Read the model definition and answer for the solid it produces. Units are mm, in the model's axes. Coordinates: 2 decimals unless noted, no trailing zeros. Order: outer loops, then holes, each group sorted by start corner. A loop starts at its lowest first (then second) coordinate and runs counter-clockwise, first axis right, second up. Notation, with made-up numbers: (-8.5, -25) -> (-2.5, -25) arc R35 ccw to (-2.5, 10) -> close; hole circle Ø4 at (39, -27). An arc over 180 degrees is marked (long way). Answer as a JSON object with one key per item and string values. Group by question number.
1) Section A-A on x = -12.5 is taken. Determine the outline of the cut face in (y, z), and give its area (4 significant figures).
2) Section C-C on y = 60 is taken. Determine the outline of the cut face in (x, z), and give its area (3 significant figures).
3) Consider L1, parallel to Y at x = 41, z = 0; L2, parallel to Y at x = -4, z = -0.75; L3, parallel to X at y = 7, z = 0.75. Determine where each line is inside the solid, lowest interval first.
4) Section B-B on y = 30 is taken. Determine the outline of the cut face in (x, z).
5) Section D-D on z = -0.5 is taken. Count the separate pieces of the cut face and the enclosed holes in it, and give its area (3 significant figures).
6) Given pin 1 (4 mm diameter, centred on x = -4, y = 4, fed in from +Z), flat-ended and moving along its own axis, determine where the tip first touches the part or whether it passes through.
7) Determine the mould class of faces 1 (the flat face through (-1, 0, 0)), 2 (the cylindrical face through (-2.17, 50.24, 0.07)), 3 (the flat face through (60, 59, 0)) for opening direction Y: released by +Y, released by -Y, zero draft, split by the parting line, or undercut.
from build123d import *

# Parameters (mm, degrees)
SKETCH1_W           = 120
SKETCH1_H           = 10
BOSS_EXTRUDE1_DEPTH = 120
SKETCH2_R           = 2.25
SKETCH2_R_2         = 2.75
SKETCH2_R_3         = 10
SKETCH2_R_4         = 3.25
CUT_EXTRUDE1_DEPTH  = 10


with BuildPart() as part:
    # Sketch1 → Boss-Extrude1 (new body)
    with BuildSketch(Plane(origin=(0, 0, 0), x_dir=(1, 0, 0), z_dir=(0, 1, 0))):
        Rectangle(SKETCH1_W, SKETCH1_H)
    extrude(amount=BOSS_EXTRUDE1_DEPTH)

    # Sketch2 → Cut-Extrude1 (cut)
    with BuildSketch(Plane.XY.offset(5)):
        with Locations((-17.5, 77.5)):
            Circle(SKETCH2_R)
        with Locations((-12.5, 47.5)):
            Circle(SKETCH2_R)
        with Locations((12.5, 47.5)):
            Circle(SKETCH2_R)
        with Locations((17.5, 77.5)):
            Circle(SKETCH2_R)
        with Locations((55, 5)):
            Circle(SKETCH2_R_2)
        with Locations((55, 115)):
            Circle(SKETCH2_R_2)
        with Locations((0, 60)):
            Circle(SKETCH2_R_3)
        with Locations((-41, 90)):
            Circle(SKETCH2_R_2)
        with Locations((-41, 60)):
            Circle(SKETCH2_R_2)
        with Locations((-41, 30)):
            Circle(SKETCH2_R_2)
        with Locations((41, 30)):
            Circle(SKETCH2_R_2)
        with Locations((41, 60)):
            Circle(SKETCH2_R_2)
        with Locations((-4, 116)):
            Circle(SKETCH2_R_4)
        with Locations((4, 116)):
            Circle(SKETCH2_R_4)
        with Locations((41, 90)):
            Circle(SKETCH2_R_2)
        with Locations((-4, 4)):
            Circle(SKETCH2_R_4)
        with Locations((4, 4)):
            Circle(SKETCH2_R_4)
        with Locations((-55, 5)):
            Circle(SKETCH2_R_2)
        with Locations((-55, 115)):
            Circle(SKETCH2_R_2)
    extrude(amount=-CUT_EXTRUDE1_DEPTH, mode=Mode.SUBTRACT)


solid = part.part
Worked answers:
{
 "1": {"outline": "(0, -5) -> (45.25, -5) -> (45.25, 5) -> (0, 5) -> close; (49.75, -5) -> (120, -5) -> (120, 5) -> (49.75, 5) -> close", "area": "1,155 mm²"},
 "2": {"outline": "(-60, -5) -> (-43.75, -5) -> (-43.75, 5) -> (-60, 5) -> close; (-38.25, -5) -> (-10, -5) -> (-10, 5) -> (-38.25, 5) -> close; (10, -5) -> (38.25, -5) -> (38.25, 5) -> (10, 5) -> close; (43.75, -5) -> (60, -5) -> (60, 5) -> (43.75, 5) -> close", "area": "890 mm²"},
 "3": {"L1": "y = 0 to 27.25, 32.75 to 57.25, 62.75 to 87.25, 92.75 to 120", "L2": "y = 0 to 0.75, 7.25 to 50.83, 69.17 to 112.75, 119.25 to 120", "L3": "x = -60 to -56.89, -53.11 to -5.25, -2.75 to 2.75, 5.25 to 53.11, 56.89 to 60"},
 "4": {"outline": "(-60, -5) -> (-43.75, -5) -> (-43.75, 5) -> (-60, 5) -> close; (-38.25, -5) -> (38.25, -5) -> (38.25, 5) -> (-38.25, 5) -> close; (43.75, -5) -> (60, -5) -> (60, 5) -> (43.75, 5) -> close"},
 "5": {"separate pieces": "1", "enclosed holes": "19", "area": "13,700 mm²"},
 "6": {"pin 1": "passes through"},
 "7": {"face 1": "released by -Y", "face 2": "undercut", "face 3": "zero draft"}
}
